Autodesk Inventor part; units mm, degrees
ref_plane "YZ Plane" through (0, 0, 0) normal (1, 0, 0) x (0, 1, 0)
ref_plane "XZ Plane" through (0, 0, 0) normal (0, 1, 0) x (-1, 0, 0)
ref_plane "XY Plane" through (0, 0, 0) normal (0, 0, 1) x (1, 0, 0)
sketch "Sketch1" plane through (0, 0, 0) normal (0, 1, 0) x (-1, 0, 0)
  line L0 (6, 0) -> (110, 0)
  line L1 (110, 0) -> (110, -104)
  line L2 (104, -110) -> (0, -110)
  line L3 (0, -110) -> (0, -6)
  arc A0 (104, -110) -> (110, -104) centre (104, -104) ccw
  arc A1 (6, 0) -> (0, -6) centre (6, -6) ccw
  point P0 (0, 0)
  point P1 (110, -110)
  dimension "d0" = 110
  dimension "d1" = 110
  dimension "d2" = 6
extrude "Extrusion1" add sketch "Sketch1" along normal blind 3
fillet "Fillet1" radius 6 2 edges at (-110, 1.5, 0) (0, 1.5, -110)
sketch "Sketch2" plane through (0, 3, 0) normal (0, 1, 0) x (1, 0, 0)
  line L0 (-88, 75) -> (-101, 75)
  line L1 (-101, 75) -> (-101, 89)
  line L2 (-101, 89) -> (-88, 89)
  line L3 (-88, 89) -> (-88, 75)
  line L4 (-6, 110) -> (-104, 110)
  line L5 (-110, 104) -> (-110, 6)
  line L6 (-101, 38) -> (-97, 38)
  line L7 (-97, 38) -> (-97, 73)
  line L8 (-97, 73) -> (-101, 73)
  line L9 (-101, 73) -> (-101, 38)
  circle A0 centre (-55, 89) radius 3.25
  circle A1 centre (-95, 15) radius 5.5
  line L10 (-104, 0) -> (-6, 0)
  circle A2 centre (-55, 15) radius 7
  line L11 (0, 6) -> (0, 104)
  point P0 (0, 0)
  point P1 (-94.5, 89)
  point P2 (-99, 73)
  point P3 (-99, 38)
  dimension "d6" = 21
  dimension "d7" = 14
  dimension "d8" = 9
  dimension "d11" = 13
  dimension "d12" = 4
  dimension "d13" = 35
  dimension "d14" = 9
  dimension "d15" = 2
  dimension "d55" = 6.5
  dimension "d56" = 55
  dimension "d57" = 21
  dimension "d58" = 11
  dimension "d59" = 15
  dimension "d60" = 15
  dimension "d61" = 14
  dimension "d62" = 15
  dimension "d63" = 55
extrude "Extrusion2" cut sketch "Sketch2" against normal blind 3
sketch "Sketch3" plane through (0, 0, 0) normal (0, -1, 0) x (1, 0, 0)
  line L0 (-88, -106.5) -> (-96, -106.5)
  line L1 (-96, -106.5) -> (-96, -104)
  line L2 (-96, -104) -> (-88, -104)
  line L3 (-88, -104) -> (-88, -106.5)
  line L4 (-6, -110) -> (-104, -110)
  line L5 (-110, -104) -> (-110, -6)
  line L6 (-14, -106.5) -> (-22, -106.5)
  line L7 (-22, -106.5) -> (-22, -104)
  line L8 (-22, -104) -> (-14, -104)
  line L9 (-14, -104) -> (-14, -106.5)
  line L10 (-88, -6) -> (-96, -6)
  line L11 (-96, -6) -> (-96, -3.5)
  line L12 (-96, -3.5) -> (-88, -3.5)
  line L13 (-88, -3.5) -> (-88, -6)
  line L14 (-14, -6) -> (-22, -6)
  line L15 (-22, -6) -> (-22, -3.5)
  line L16 (-22, -3.5) -> (-14, -3.5)
  line L17 (-14, -3.5) -> (-14, -6)
  line L18 (-104, -14) -> (-106.5, -14)
  line L19 (-106.5, -14) -> (-106.5, -22)
  line L20 (-106.5, -22) -> (-104, -22)
  line L21 (-104, -22) -> (-104, -14)
  line L22 (-104, 0) -> (-6, 0)
  line L23 (-104, -96) -> (-104, -88)
  line L24 (-104, -88) -> (-106.5, -88)
  line L25 (-106.5, -88) -> (-106.5, -96)
  line L26 (-106.5, -96) -> (-104, -96)
  line L27 (-3.5, -22) -> (-3.5, -14)
  line L28 (-3.5, -14) -> (-6, -14)
  line L29 (-6, -14) -> (-6, -22)
  line L30 (-6, -22) -> (-3.5, -22)
  line L31 (-3.5, -96) -> (-3.5, -88)
  line L32 (-3.5, -88) -> (-6, -88)
  line L33 (-6, -88) -> (-6, -96)
  line L34 (-6, -96) -> (-3.5, -96)
  point P0 (0, 0)
  dimension "d20" = 8
  dimension "d21" = 2.5
  dimension "d22" = 3.5
  dimension "d23" = 14
  dimension "d26" = 74
  dimension "d29" = 100.5
  dimension "d67" = 8
  dimension "d68" = 2.5
  dimension "d69" = 3.5
  dimension "d70" = 14
  dimension "d73" = 74
  dimension "d76" = 100.5
extrude "Extrusion3" add sketch "Sketch3" along normal blind 8.1
sketch "Sketch4" plane through (-88, 0, -106.5) normal (0, 0, -1) x (-1, 0, 0)
  line L0 (0, 0) -> (0, -8.1)
  line L1 (8, -8.1) -> (0, -8.1)
  line L2 (0, -8.1) -> (0, -4.1)
  line L3 (0, -4.1) -> (8, -4.1)
  line L4 (8, -4.1) -> (8, -8.1)
  line L5 (8, -8.1) -> (0, -8.1)
  line L6 (8, 0) -> (8, -8.1)
  line L7 (-66, 0) -> (-66, -8.1)
  line L8 (-74, 0) -> (-74, -8.1)
  line L9 (-66, -8.1) -> (-74, -8.1)
  line L10 (-74, -8.1) -> (-74, -4.1)
  line L11 (-74, -4.1) -> (-66, -4.1)
  line L12 (-66, -4.1) -> (-66, -8.1)
  point P0 (-88, 0)
  point P1 (0, -8.1)
  dimension "d34" = 4
  dimension "d35" = 0
  dimension "d36" = 0
  dimension "d37" = 4
extrude "Extrusion4" add sketch "Sketch4" along normal blind 2
chamfer "Chamfer1" distance 3 angle 45 2 edges at (-92, -8.1, -108.5) (-18, -8.1, -108.5)
fillet "Fillet2" radius 1 6 edges at (-92, -5.1, -108.5) (-18, -5.1, -108.5) (-18, -8.1, -105.5) (-92, -8.1, -105.5) (-92, -8.1, -104) (-18, -8.1, -104)
fillet "Fillet3" radius 0.5 2 edges at (-92, -4.1, -108.5) (-18, -4.1, -108.5)
sketch "Sketch5" plane through (-96, 0, -3.5) normal (0, 0, 1) x (1, 0, 0)
  line L0 (8, 0) -> (8, -8.1)
  line L1 (0, 0) -> (0, -8.1)
  line L2 (8, -8.1) -> (0, -8.1)
  line L3 (0, -8.1) -> (0, -4.05)
  line L4 (0, -4.05) -> (8, -4.05)
  line L5 (8, -4.05) -> (8, -8.1)
  line L6 (82, -8.1) -> (74, -8.1)
  line L7 (82, -8.1) -> (74, -8.1)
  line L8 (74, -8.1) -> (74, -4.1)
  line L9 (74, -4.1) -> (82, -4.1)
  line L10 (82, -4.1) -> (82, -8.1)
  point P0 (96, 0)
  point P1 (8, -4.05)
  dimension "d45" = 4.05
extrude "Extrusion5" add sketch "Sketch5" along normal blind 2
chamfer "Chamfer2" distance 3 angle 45 2 edges at (-92, -8.1, -1.5) (-18, -8.1, -1.5)
fillet "Fillet4" radius 1 6 edges at (-18, -8.1, -4.5) (-18, -5.1, -1.5) (-18, -8.1, -6) (-92, -8.1, -4.5) (-92, -5.1, -1.5) (-92, -8.1, -6)
fillet "Fillet5" radius 0.5 2 edges at (-92, -4.05, -1.5) (-18, -4.1, -1.5)
fillet "Fillet6" radius 1 1 edges at (-92, 0, -104)
fillet "Fillet7" radius 1 3 edges at (-18, 0, -104) (-18, 0, -6) (-92, 0, -6)
sketch "Sketch6" plane through (0, 0, 0) normal (0, -1, 0) x (1, 0, 0)
  circle A0 centre (-55, -15) radius 7
  circle A1 centre (-55, -15) radius 9
  point P0 (0, 0)
  dimension "d64" = 18
extrude "Extrusion6" cut sketch "Sketch6" against normal blind 1.2 contours A0 | A1
sketch "Sketch7" plane through (0, -8.1, 0) normal (0, -1, 0) x (1, 0, 0)
  line L0 (-106.5, -14) -> (-106.5, -22)
  line L1 (-104, -22) -> (-104, -14)
  line L2 (-106.5, -14) -> (-104, -14)
  line L3 (-104, -14) -> (-104, -22)
  line L4 (-104, -22) -> (-106.5, -22)
  line L5 (-106.5, -22) -> (-106.5, -14)
  line L6 (-104, -88) -> (-106.5, -88)
  line L7 (-106.5, -88) -> (-104, -88)
  line L8 (-104, -88) -> (-104, -96)
  line L9 (-104, -96) -> (-106.5, -96)
  line L10 (-106.5, -96) -> (-106.5, -88)
  line L11 (-6, -22) -> (-6, -14)
  line L12 (-3.5, -14) -> (-3.5, -22)
  line L13 (-6, -14) -> (-3.5, -14)
  line L14 (-3.5, -14) -> (-3.5, -22)
  line L15 (-3.5, -22) -> (-6, -22)
  line L16 (-6, -22) -> (-6, -14)
  line L17 (-6, -88) -> (-3.5, -88)
  line L18 (-3.5, -96) -> (-6, -96)
  line L19 (-6, -88) -> (-3.5, -88)
  line L20 (-3.5, -88) -> (-3.5, -96)
  line L21 (-3.5, -96) -> (-6, -96)
  line L22 (-6, -96) -> (-6, -88)
  point P0 (0, 0)
  dimension "d81" = 8
extrude "Extrusion7" cut sketch "Sketch7" against normal blind 5
chamfer "Chamfer3" distance 1 angle 45 4 edges at (-3.5, -3.1, -92) (-3.5, -3.1, -18) (-106.5, -3.1, -92) (-106.5, -3.1, -18)
equation "\"d14\" = d8"
equation "\"d56\" = 0.5 * d0"
equation "\"d57\" = d6"
equation "\"d63\" = 0.5 * d0"
equation "\"d26\" = d0 - d20 - 2 * d23"
equation "\"d29\" = d1 - d21 - 2 * d22"
equation "\"d67\" = d20"
equation "\"d68\" = d21"
equation "\"d69\" = d22"
equation "\"d70\" = d23"
equation "\"d73\" = d26"
equation "\"d76\" = d29"
properties part number "Cover-USB side"
The listing builds one solid part. Answer for the finished solid, in the listing's coordinates (mm). A direction names the side the tool comes from. Give positions to 0.01 mm unless a question says otherwise; leave off trailing zeros. Write each loop counter-clockwise with the first axis right and the second up, starting at its lowest first coordinate (ties: lowest second). Pieces come first, ordered by that corner, then holes. Notation, with made-up numbers: (-10, 43) -> (42, 43) arc R18 cw to (42, 47) -> close; hole circle Ø10 at (4.25, 83). An arc over 180 degrees is marked (long way). Use one line per item in the form item = value.
1) Straight lines are drawn through the part: probe 1 along X at (y, z) = (2.45, -15); probe 2 along Z at (x, y) = (-55, 0.8); probe 3 along X at (y, z) = (-0.25, -21). For each, find the intervals that lie inside material, in ascending order.
Result:
probe_1 = -110 to -100.5, -89.5 to -62, -48 to 0
probe_2 = -110 to -92.25, -85.75 to -24, -6 to 0
probe_3 = -106.5 to -104, -6 to -3.5
2) Section C-C on x = -68.5 is taken. Write down the section's boundary in (y, z), plus the area to 3 significant figures.
Result:
outline = (0, -110) -> (3, -110) -> (3, 0) -> (0, 0) -> close
area = 330 mm²
3) Each of these flat-tipped pins is pushed along its axis until it touches: P1, Ø6, axis at y = -4, z = -4.5, coming from the +X side; P2, Ø4.5, axis at y = -6, z = -106, coming from the -X side; P3, Ø1, axis at x = -16, y = -5.5, coming from the +Z side. Where does it stop, or does it pass through?
Result:
P1 = -14
P2 = -96
P3 = -1.55
4) For a pull along X with two mould halves and no side action, classify faces 6 (the flat face through (-17.9, -6.6, -107)), 7 (the flat face through (-96, -4, -106)), 8 (the flat face through (-55, 1.2, -22.3)), 9 (the flat face through (-104, -2, -18)) as +X half, -X half, draft (parallel to the pull), parting line (faces both ways), or undercut.
Result:
face_6 = draft
face_7 = -X half
face_8 = undercut
face_9 = undercut
5) Section A-A on x = -55 is taken. Write down the section's boundary in (y, z), plus the area to 3 significant figures.
Result:
outline = (0, -110) -> (3, -110) -> (3, -92.25) -> (0, -92.25) -> close; (0, -85.75) -> (3, -85.75) -> (3, -22) -> (1.2, -22) -> (1.2, -24) -> (0, -24) -> close; (0, -6) -> (1.2, -6) -> (1.2, -8) -> (3, -8) -> (3, 0) -> (0, 0) -> close
area = 264 mm²
6) Section B-B on z = -82 is taken. Write down the section's boundary in (x, y), plus the area to 3 significant figures.
Result:
outline = (-110, 0) -> (-101, 0) -> (-101, 3) -> (-110, 3) -> close; (-88, 0) -> (0, 0) -> (0, 3) -> (-88, 3) -> close
area = 291 mm²
7) A tool of negligible diameter and unlimited length cuts with its end or side. For faces 1 (the flat face through (-18, -2, -106.5)), 2 (the flat face through (-88, 2, -82)), 3 (the flat face through (-14, -4, -4)), 4 (the flat face through (-104, -2, -92)), 5 (the flat face through (-92, -4, -6)), from which of +Z, -Z, +X, -X, +Y, -Y can it reach the whole face along a straight path? Write none if from no direction.
Result:
face_1 = -Z, +X, -X
face_2 = +Y, -Y
face_3 = +Z, -Z, +X, -Y
face_4 = +Z, -Z, -Y
face_5 = +X, -X, -Y
